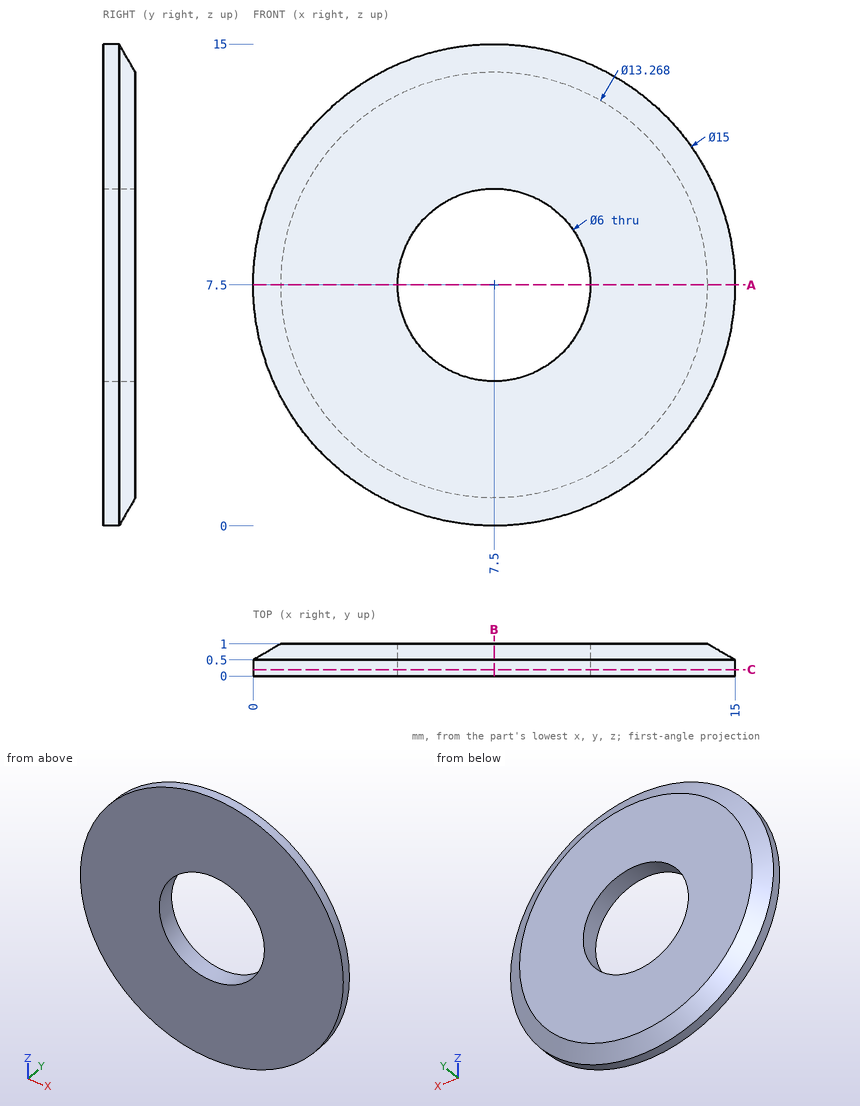
Source: three-view drawing plus pictorial views. Frame: mm from the lowest corner of the part. Give positions to 0.01 mm unless a question says otherwise; leave off trailing zeros. Loops run counter-clockwise (first coordinate to the right, second up) from the corner with the lowest first, then second, coordinate; pieces in that order, holes last. Notation, with made-up numbers: (87, -33.75) -> (122, -33.75) arc R22 ccw to (122, -18.75) -> close; hole circle Ø11 at (83, 23.25). An arc over 180 degrees is marked (long way). Use a Markdown table: item, result. Add a question column.
(1) Section query B-B (x = 7.5). Output: boundary loops of the cut face in (y, z).
(2) First-contact query: pin 1 Ø5.5 at (x, z) = (7.5, 7.5) entering from -Y. Flat tip, straight axial feed; report the tip coordinate or a pass-through.
(3) Ray query, line 1 (X direction, y = 0.4, z = 7.5); line 2 (X direction, y = 0.8, z = 8.25) (1 decimal); line 3 (Z direction, x = 5.5, y = 0.3). Return the intervals inside material, ascending.
(4) Section query A-A (z = 7.5). Output: boundary loops of the cut face in (x, y).
(5) Section query C-C (y = 0.2). Output: boundary loops of the cut face in (x, z).
Checked values:
| question | item | result |
|---|---|---|
| 1 | outline | (0, 0) -> (0.5, 0) -> (1, 0.87) -> (1, 4.5) -> (0, 4.5) -> close; (0, 10.5) -> (1, 10.5) -> (1, 14.13) -> (0.5, 15) -> (0, 15) -> close |
| 2 | pin 1 | through |
| 3 | line 1 | 0 to 4.5, 10.5 to 15 |
| 3 | line 2 | 0.6 to 4.6, 10.4 to 14.4 |
| 3 | line 3 | 0.27 to 5.26, 9.74 to 14.73 |
| 4 | outline | (0, 0) -> (4.5, 0) -> (4.5, 1) -> (0.87, 1) -> (0, 0.5) -> close; (10.5, 0) -> (15, 0) -> (15, 0.5) -> (14.13, 1) -> (10.5, 1) -> close |
| 5 | outline | circle Ø15 at (7.5, 7.5); hole circle Ø6 at (7.5, 7.5) |
